Can you work these out from the model? Positions are in its coordinate system, mm. Give positions to 0.01 mm unless a question says otherwise; leave off trailing zeros. Loops run counter-clockwise (first coordinate to the right, second up) from the corner with the lowest first, then second, coordinate; pieces in that order, holes last. Notation, with made-up numbers: (2.25, 39.5) - (31.25, 39.5) arc R31 cw to (31.25, 69.5) - close; hole circle Ø9 at (39.25, 23). An arc over 180 degrees is marked (long way). Answer as a JSON object with one key per item and string values. Group by question number.
Item 1: Suppose I cut it at C-C on x = 10. Write out the boundary of the cut face in (y, z), and give its area (3 significant figures).
Item 2: Suppose I cut it at A-A on z = 0. Write out the boundary of the cut face in (x, y).
Item 3: Will this pin go through, and if not, where does the flat tip stop? pin 1 (3 mm diameter, centred on x = 0, z = 0, fed in from +Y).
Item 4: Suppose I cut it at B-B on y = 1.1. Write out the boundary of the cut face in (x, z), and give its area (3 significant figures).
Item 5: Please list where these lines run through material, in increasing order: L1, parallel to X at y = 0.1, z = 0; L2, parallel to X at y = 0.75, z = 0; L3, parallel to Z at x = 0, y = 0.35.
Item 6: Thinking about a two-plate mould opening in X: for faces 1 (the cylindrical face through (-0.91, 0.3, 0.7)), 2 (the flat face through (8, 0, 0)), 3 (the flat face through (9.03, 0.89, 2.74)), which applies, pulls with the +X half, pulls with the -X half, needs draft (parallel to the pull), parting line crosses it, or undercut?
from build123d import *

# Parameters (mm, degrees)
SKETCH_1_R      = 1.15
SKETCH_1_R_2    = 0.9
EXTRUDE_1_DEPTH = 1.8
CHAMFER_1_SIZE  = 1.2


with BuildPart() as part:
    # Эскиз1 → Бобышка-Вытянуть1 (new body)
    with BuildSketch(Plane(origin=(0, 0, 0), x_dir=(1, 0, 0), z_dir=(0, 1, 0))):
        with BuildLine():
            Line((0.185714286, 3.244689539), (17.628571429, 2.246323527))
            ThreePointArc((17.628571429, 2.246323527), (19.75, 0), (17.628571429, -2.246323527))
            Line((17.628571429, -2.246323527), (0.185714286, -3.244689539))
            ThreePointArc((0.185714286, -3.244689539), (-3.25, 0), (0.185714286, 3.244689539))
        make_face()
        Circle(SKETCH_1_R, mode=Mode.SUBTRACT)
        with Locations((17.5, 0)):
            Circle(SKETCH_1_R_2, mode=Mode.SUBTRACT)
    extrude(amount=EXTRUDE_1_DEPTH)

    # Фаска1
    chamfer_1_edges = [part.edges().sort_by_distance(p)[0] for p in [
        (-1.15, 1.8, 0),
    ]]
    chamfer(chamfer_1_edges, length=CHAMFER_1_SIZE)


solid = part.part
Worked out:
{
 "1": {"outline": "(0, -2.68) - (1.8, -2.68) - (1.8, 2.68) - (0, 2.68) - close", "area": "9.66 mm2"},
 "2": {"outline": "(-3.25, 0) - (-1.15, 0) - (-1.15, 0.6) - (-2.35, 1.8) - (-3.25, 1.8) - close; (1.15, 0) - (16.6, 0) - (16.6, 1.8) - (2.35, 1.8) - (1.15, 0.6) - close; (18.4, 0) - (19.75, 0) - (19.75, 1.8) - (18.4, 1.8) - close"},
 "3": {"pin 1": "stops at y = 0.95"},
 "4": {"outline": "(0.19, -3.24) - (17.63, -2.25) arc R2.25 ccw to (17.63, 2.25) - (0.19, 3.24) arc R3.25 ccw (long way) to start; hole circle Ø3.3 at (0, 0); hole circle Ø1.8 at (17.5, 0)", "area": "110 mm2"},
 "5": {"L1": "x = -3.25 to -1.15, 1.15 to 16.6, 18.4 to 19.75", "L2": "x = -3.25 to -1.3, 1.3 to 16.6, 18.4 to 19.75", "L3": "z = -3.25 to -1.15, 1.15 to 3.25"},
 "6": {"face 1": "undercut", "face 2": "needs draft", "face 3": "pulls with the +X half"}
}
